Verification items for the finished model (mm, model axes). Give positions to 0.01 mm unless a question says otherwise; leave off trailing zeros. Loops run counter-clockwise (first coordinate to the right, second up) from the corner with the lowest first, then second, coordinate; pieces in that order, holes last. Notation, with made-up numbers: (5.5, 79.5) - (61.5, 79.5) arc R17 cw to (61.5, 95.5) - close; hole circle Ø3 at (66, 3.5). An arc over 180 degrees is marked (long way). One line per item, written item: value. Start each with the question number.
1. Sectioned sample at A-A (y = 2.1). Count the separate pieces of the cut face and the enclosed holes in it, plus the area to 3 significant figures.
2. Scan lines: L1, parallel to Z at x = 15.5, y = 2.5; L2, parallel to Z at x = -2, y = 1.2; L3, parallel to X at y = 1.5, z = -15. Record each from-to range of solid material in increasing order. Write a range as [from, to].
3. Sectioned sample at C-C (x = -15.5). Record the cut outline in (y, z) (3 decimals).
4. Gauge pin test, flat end, axial feed: pin 1 (1 mm diameter, centred on y = 1, z = -7, fed in from -X). Record the tip position at first contact, or that the pin passes through.
5. Sectioned sample at B-B (z = -22.5). Record the cut outline in (x, y) (3 decimals).
6. Sectioned sample at D-D (z = -15.5). Record the cut outline in (x, y) (3 decimals).
from build123d import *

# Parameters (mm, degrees)
SKETCH1_R                 = 28.063300378
BOSS_EXTRUDE1_DEPTH       = 3.175
M3X0_5_TAPPED_HOLE1_D     = 2.5
M3X0_5_TAPPED_HOLE1_DEPTH = 7.62
M3X0_5_TAPPED_HOLE1_TIP   = 0.751075774
SKETCH5_R                 = 2.38125
CUT_EXTRUDE1_DEPTH        = 40.814297448
CIRPATTERN1_COUNT         = 4


with BuildPart() as part:
    # Sketch1 → Boss-Extrude1 (new body)
    with BuildSketch(Plane(origin=(0, 0, 0), x_dir=(1, 0, 0), z_dir=(0, 1, 0))):
        with Locations(Location((0, 0, 0), (0, 0, 270))):
            Circle(SKETCH1_R)
    extrude(amount=BOSS_EXTRUDE1_DEPTH)

    # M3x0.5 Tapped Hole1
    with Locations(Plane(origin=(0, 3.175, 0), x_dir=(1, 0, 0), z_dir=(0, 1, 0))):
        with Locations((-15.5, 15.5), (15.5, -15.5), (15.5, 15.5), (-15.5, -15.5)):
            Hole(M3X0_5_TAPPED_HOLE1_D / 2, depth=M3X0_5_TAPPED_HOLE1_DEPTH)
            with Locations((0, 0, -(M3X0_5_TAPPED_HOLE1_DEPTH + M3X0_5_TAPPED_HOLE1_TIP / 2))):  # 118° drill point
                Cone(0, M3X0_5_TAPPED_HOLE1_D / 2, M3X0_5_TAPPED_HOLE1_TIP, mode=Mode.SUBTRACT)

    # Sketch5 → Cut-Extrude1 (cut, through all)
    with BuildSketch(Plane(origin=(0, 3.175, 0), x_dir=(1, 0, 0), z_dir=(0, 1, 0))):
        with Locations(Location((0, 23.8125, 0), (0, 0, 270))):
            Circle(SKETCH5_R)
    cut_extrude1 = extrude(amount=-CUT_EXTRUDE1_DEPTH, mode=Mode.SUBTRACT)

    # CirPattern1: Cut-Extrude1 ×4 about axis
    cirpattern1_axis = Axis((0, 0, 0), (0, 1, 0))
    for i in range(1, CIRPATTERN1_COUNT):
        add(cut_extrude1.rotate(cirpattern1_axis, i * 360 / CIRPATTERN1_COUNT), mode=Mode.SUBTRACT)


solid = part.part
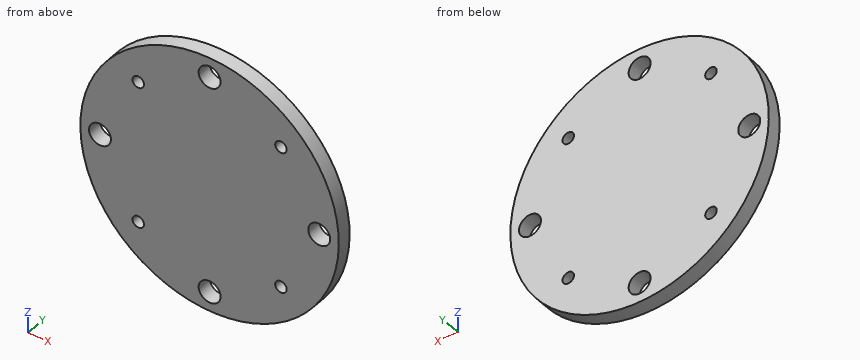
Results are:
1. separate pieces: 1
1. enclosed holes: 8
1. area: 2,380 mm^2
2. L1: z = [-23.39, -16.75], [-14.25, 14.25], [16.75, 23.39]
2. L2: z = [-27.99, -25.1], [-22.52, 22.52], [25.1, 27.99]
2. L3: x = [-23.72, -16.65], [-14.35, 14.35], [16.65, 23.72]
3. outline: (0, -23.394) - (3.175, -23.394) - (3.175, -16.75) - (0, -16.75) - close; (0, -14.25) - (3.175, -14.25) - (3.175, 14.25) - (0, 14.25) - close; (0, 16.75) - (3.175, 16.75) - (3.175, 23.394) - (0, 23.394) - close
4. pin 1: stops at x = -27.3
5. outline: (-16.772, 0) - (-1.987, 0) - (-1.987, 3.175) - (-16.772, 3.175) - close; (1.987, 0) - (16.772, 0) - (16.772, 3.175) - (1.987, 3.175) - close
6. outline: (-23.394, 0) - (-16.75, 0) - (-16.75, 3.175) - (-23.394, 3.175) - close; (-14.25, 0) - (14.25, 0) - (14.25, 3.175) - (-14.25, 3.175) - close; (16.75, 0) - (23.394, 0) - (23.394, 3.175) - (16.75, 3.175) - close
